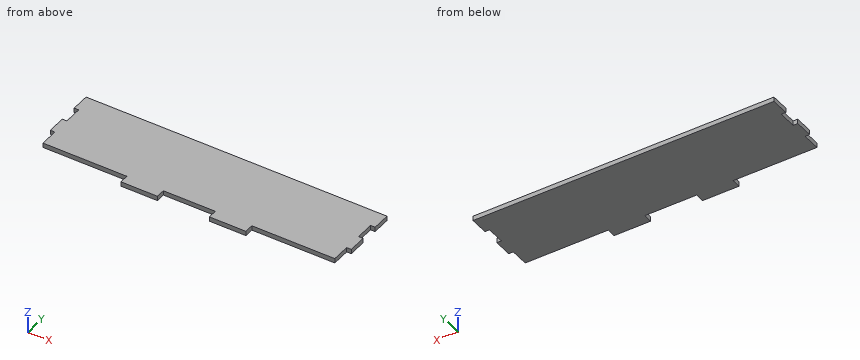
from build123d import *

# Parameters (mm, degrees)
SKETCH1_W           = 203.2
SKETCH1_H           = 101.6
BOSS_EXTRUDE1_DEPTH = 3.175
SKETCH2_W           = 3.175
SKETCH2_H           = 12.7
SKETCH2_W_2         = 25.4
SKETCH2_H_2         = 6.35
BOSS_EXTRUDE2_DEPTH = 3.175
SKETCH3_W           = 25.4
SKETCH3_H           = 6.35
CUT_EXTRUDE1_DEPTH  = 120.947785411
SKETCH4_W           = 245.475029748
SKETCH4_H           = 66.468196642
CUT_EXTRUDE2_DEPTH  = 120.390132549


with BuildPart() as part:
    # Sketch1 → Boss-Extrude1 (new body)
    with BuildSketch(Plane.XY):
        Rectangle(SKETCH1_W, SKETCH1_H)
    extrude(amount=BOSS_EXTRUDE1_DEPTH)

    # Sketch2 → Boss-Extrude2 (add)
    with BuildSketch(Plane.XY.offset(3.175)):
        with Locations((-103.1875, 19.05)):
            Rectangle(SKETCH2_W, SKETCH2_H)
        with Locations((-103.1875, 44.45)):
            Rectangle(SKETCH2_W, SKETCH2_H)
        with Locations((-103.1875, -6.35)):
            Rectangle(SKETCH2_W, SKETCH2_H)
        with Locations((-103.1875, -31.75)):
            Rectangle(SKETCH2_W, SKETCH2_H)
        with Locations((-92.075, -53.975)):
            Rectangle(SKETCH2_W_2, SKETCH2_H_2)
        with Locations((-30.48, -53.975)):
            Rectangle(SKETCH2_W_2, SKETCH2_H_2)
        with Locations((31.115, -53.975)):
            Rectangle(SKETCH2_W_2, SKETCH2_H_2)
        with Locations((92.71, -53.975)):
            Rectangle(SKETCH2_W_2, SKETCH2_H_2)
        with Locations((103.1875, -31.75)):
            Rectangle(SKETCH2_W, SKETCH2_H)
        with Locations((103.1875, -6.35)):
            Rectangle(SKETCH2_W, SKETCH2_H)
        with Locations((103.1875, 19.05)):
            Rectangle(SKETCH2_W, SKETCH2_H)
        with Locations((103.1875, 44.45)):
            Rectangle(SKETCH2_W, SKETCH2_H)
    extrude(amount=-BOSS_EXTRUDE2_DEPTH)

    # Sketch3 → Cut-Extrude1 (cut, through all)
    with BuildSketch(Plane.XY.offset(3.175)):
        with Locations((-92.075, -53.975)):
            Rectangle(SKETCH3_W, SKETCH3_H)
        with Locations((92.71, -53.975)):
            Rectangle(SKETCH3_W, SKETCH3_H)
    extrude(amount=-CUT_EXTRUDE1_DEPTH, mode=Mode.SUBTRACT)

    # Sketch4 → Cut-Extrude2 (cut, through all)
    with BuildSketch(Plane.XY.offset(3.175)):
        with Locations((-8.102055055, 33.234098321)):
            Rectangle(SKETCH4_W, SKETCH4_H)
    extrude(amount=-CUT_EXTRUDE2_DEPTH, mode=Mode.SUBTRACT)


solid = part.part
Could you check a few things on this model? Use its own coordinates, in mm. Coordinates: 2 decimals unless noted, no trailing zeros. Loops run counter-clockwise (first coordinate to the right, second up) from the corner with the lowest first, then second, coordinate; pieces in that order, holes last.
1. I need wall thicknesses on L1, parallel to X at y = -53, z = 2.8 (3 decimals); L2, parallel to Y at x = 49, z = 2.95; L3, parallel to X at y = -14, z = 1.1. Which ranges of each line are inside material? Lowest first, please.
2. For P1, Ø2, axis at x = 36, y = -38, coming from the -Z side; P2, Ø1, axis at y = -15, z = 2, coming from the +X side; P3, Ø1, axis at y = -54.5, z = 2, coming from the +X side (3 decimals); P4, Ø1, axis at y = -53.5, z = 1, coming from the -X side, each with a flat end and sliding along its axis, tell me the tip position at first contact or that it passes through.
3. Imagine slicing it at C-C (y = -19). Please give me the cut outline in (x, z) (3 decimals), and give its area (3 significant figures).
4. Imagine slicing it at A-A (z = 0.5). Please give me the cut outline in (x, y) (3 decimals).
5. Imagine slicing it at B-B (x = 64). Please give me the cut outline in (y, z) (3 decimals), and give its area (3 significant figures).
Computed values:
1. L1: x = -43.18 to -17.78, 18.415 to 43.815
1. L2: y = -50.8 to 0
1. L3: x = -101.6 to 101.6
2. P1: stops at z = 0
2. P2: stops at x = 101.6
2. P3: stops at x = 43.815
2. P4: stops at x = -43.18
3. outline: (-101.6, 0) - (101.6, 0) - (101.6, 3.175) - (-101.6, 3.175) - close
3. area: 645 mm2
4. outline: (-104.775, -38.1) - (-101.6, -38.1) - (-101.6, -50.8) - (-43.18, -50.8) - (-43.18, -57.15) - (-17.78, -57.15) - (-17.78, -50.8) - (18.415, -50.8) - (18.415, -57.15) - (43.815, -57.15) - (43.815, -50.8) - (101.6, -50.8) - (101.6, -38.1) - (104.775, -38.1) - (104.775, -25.4) - (101.6, -25.4) - (101.6, -12.7) - (104.775, -12.7) - (104.775, 0) - (-104.775, 0) - (-104.775, -12.7) - (-101.6, -12.7) - (-101.6, -25.4) - (-104.775, -25.4) - close
5. outline: (-50.8, 0) - (0, 0) - (0, 3.175) - (-50.8, 3.175) - close
5. area: 161 mm2
